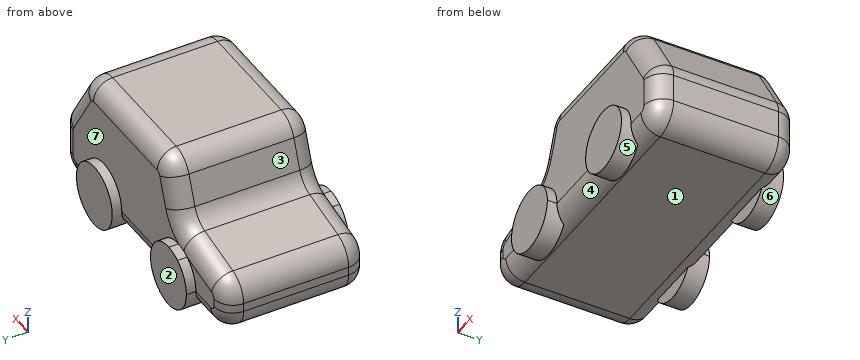
from build123d import *

# Parameters (mm, degrees)
F1_DEPTH = 19.05
F2_R     = 5.08
F4_DEPTH = 2.54


with BuildPart() as f1:
    # F0 (on Front) → F1 (new body, symmetric)
    with BuildSketch(Plane.XZ):
        with BuildLine():
            Line((-31.7947502343, 28.5244368225), (-45.0228915296, 25.7004508864))
            ThreePointArc((-45.0228915296, 25.7004508864), (-48.6337945871, 23.4843832577), (-50.0471470773, 19.4903863419))
            Line((-50.0471470773, 19.4903863419), (-50.0471470773, 17.209751375))
            ThreePointArc((-50.0471470773, 17.209751375), (-48.1872751379, 12.7196233145), (-43.6971470773, 10.859751375))
            Line((-43.6971470773, 10.859751375), (19.8028529227, 10.859751375))
            ThreePointArc((19.8028529227, 10.859751375), (24.2929809832, 12.7196233145), (26.1528529227, 17.209751375))
            Line((26.1528529227, 17.209751375), (26.1528529227, 24.5724479892))
            ThreePointArc((26.1528529227, 24.5724479892), (25.9116323119, 26.3060322456), (25.2062972144, 27.9079074459))
            Line((25.2062972144, 27.9079074459), (16.9319615885, 41.3123310901))
            ThreePointArc((16.9319615885, 41.3123310901), (14.6222474443, 43.5222601478), (11.5285172969, 44.3268716335))
            Line((11.5285172969, 44.3268716335), (-18.3973462303, 44.3268716335))
            ThreePointArc((-18.3973462303, 44.3268716335), (-22.0311174702, 43.1843860671), (-24.3573198303, 40.168039059))
            Line((-24.3573198303, 40.168039059), (-27.1605210865, 32.5433339416))
            ThreePointArc((-27.1605210865, 32.5433339416), (-28.9601695313, 29.9371901824), (-31.7947502343, 28.5244368225))
        make_face()
    extrude(amount=F1_DEPTH, both=True)

    # F2
    f2_edges = [f1.edges().sort_by_distance(p)[0] for p in [
        (-3.434414, -19.05, 44.326872),
        (-3.434414, 19.05, 44.326872),
    ]]
    fillet(f2_edges, radius=F2_R)

    # F3 (on face) → F4 (join, symmetric)
    with BuildSketch(Plane.XZ.offset(19.05)):
        with BuildLine():
            Line((15.0660514035, 15.939751375), (-1.7679906585, 15.939751375))
            ThreePointArc((-1.7679906585, 15.939751375), (6.6490303725, 7.522730344), (15.0660514035, 15.939751375))
        make_face()
        with BuildLine():
            ThreePointArc((15.0660514035, 15.939751375), (6.6490303725, 24.356772406), (-1.7679906585, 15.939751375))
            Line((-1.7679906585, 15.939751375), (15.0660514035, 15.939751375))
        make_face()
        with BuildLine():
            Line((-36.5645825066, 15.939751375), (-19.7305404446, 15.939751375))
            ThreePointArc((-19.7305404446, 15.939751375), (-22.2623397644, 21.9572598666), (-28.3346316813, 24.3546933103))
            ThreePointArc((-28.3346316813, 24.3546933103), (-29.5122474663, 23.8889745473), (-30.7341546725, 23.5563851869))
            Line((-30.7341546725, 23.5563851869), (-32.4075441475, 23.1991446466))
            ThreePointArc((-32.4075441475, 23.1991446466), (-35.451759131, 20.1224466362), (-36.5645825066, 15.939751375))
        make_face()
        with BuildLine():
            ThreePointArc((-30.7341546725, 23.5563851869), (-29.5122474663, 23.8889745473), (-28.3346316813, 24.3546933103))
            ThreePointArc((-28.3346316813, 24.3546933103), (-30.444928012, 24.0371799813), (-32.4075441475, 23.1991446466))
            Line((-32.4075441475, 23.1991446466), (-30.7341546725, 23.5563851869))
        make_face()
        with BuildLine():
            ThreePointArc((-36.5645825066, 15.939751375), (-28.1475614756, 7.522730344), (-19.7305404446, 15.939751375))
            Line((-19.7305404446, 15.939751375), (-36.5645825066, 15.939751375))
        make_face()
    extrude(amount=F4_DEPTH, both=True)

    # F5: F1 across plane


with BuildPart() as f1_1:
    add(f1.part)
    add(f1.part.mirror(Plane.XZ))


solid = f1_1.part
Work out the finished part from the listing and answer in its coordinate system (mm). Face numbers are marked on the shaded views. A direction names the side the tool comes from. Round coordinates to 2 decimals unless told otherwise and drop trailing zeros. Loops run counter-clockwise (first coordinate to the right, second up) from the corner with the lowest first, then second, coordinate; pieces in that order, holes last. Notation, with made-up numbers: (63, 20) -> (117, 20) arc R24 ccw to (117, 31) -> close; hole circle Ø10 at (72, 77). An arc over 180 degrees is marked (long way). Use one line per item in the form item = value.
(1) A tool of negligible diameter and unlimited length cuts with its end or side. For the marked faces 5, 6 and 7, from which of +Z, -Z, +X, -X, +Y, -Y can it reach the whole face along a straight path? Write none if from no direction.
Answer list:
face_5 = -Y
face_6 = +Y
face_7 = +Z, +Y
(2) Straight lines are drawn through the part: line 1 (Z direction, x = -10, y = -8.5); line 2 (Y direction, x = 9, z = 25). For each, find the intervals that lie inside material, in ascending order.
Answer list:
line_1 = 10.86 to 44.33
line_2 = -19.05 to 19.05
(3) Find section C-C on x = 9. Give the vertices of the cut face in (y, z), then the cut area to 3 significant figures.
Answer list:
outline = (-21.59, 7.86) -> (-16.51, 7.86) -> (-16.51, 11.54) arc R5.08 ccw to (-13.97, 10.86) -> (13.97, 10.86) arc R5.08 ccw to (16.51, 11.54) -> (16.51, 7.86) -> (21.59, 7.86) -> (21.59, 24.02) -> (19.05, 24.02) -> (19.05, 39.25) arc R5.08 ccw to (13.97, 44.33) -> (-13.97, 44.33) arc R5.08 ccw to (-19.05, 39.25) -> (-19.05, 24.02) -> (-21.59, 24.02) -> close
area = 1,360 mm2
(4) For a pull along Y with two mould halves and no side action, classify the marked faces 1, 2, 3 and 4 as released by +Y, released by -Y, zero draft, split by the parting line, or undercut.
Answer list:
face_1 = undercut
face_2 = released by +Y
face_3 = zero draft
face_4 = undercut
(5) Find section A-A on x = -8.5. Give the vertices of the cut face in (y, z), then the cut area to 3 significant figures.
Answer list:
outline = (-19.05, 15.94) arc R5.08 ccw to (-13.97, 10.86) -> (13.97, 10.86) arc R5.08 ccw to (19.05, 15.94) -> (19.05, 39.25) arc R5.08 ccw to (13.97, 44.33) -> (-13.97, 44.33) arc R5.08 ccw to (-19.05, 39.25) -> close
area = 1,250 mm2
(6) Flat-ended cylindrical pins translate along their axes: P1, Ø1, axis at y = 6.5, z = 14, coming from the -X side; P2, Ø2, axis at x = -37.5, z = 19.5, coming from the -Y side; P3, Ø11.5, axis at x = 7, z = 29, coming from the +Y side; P4, Ø3, axis at y = -17, z = 40, coming from the +X side. Find the tip coordinate at first contact, or state that the pin passes through.
Answer list:
P1 = -49.44
P2 = -19.05
P3 = 21.59
P4 = 17.94
(7) Find section B-B on y = -11. Give the vertices of the cut face in (x, z), then the cut area to 3 significant figures.
Answer list:
outline = (-50.05, 17.21) arc R6.35 ccw to (-43.7, 10.86) -> (19.8, 10.86) arc R6.35 ccw to (26.15, 17.21) -> (26.15, 24.57) arc R6.35 ccw to (25.21, 27.91) -> (16.93, 41.31) arc R6.35 ccw to (11.53, 44.33) -> (-18.4, 44.33) arc R6.35 ccw to (-24.36, 40.17) -> (-27.16, 32.54) arc R6.35 cw to (-31.79, 28.52) -> (-45.02, 25.7) arc R6.35 ccw to (-50.05, 19.49) -> close
area = 2,010 mm2
